Input: part model. Units: mm. Frame: model coordinates. A direction names the side the tool comes from. Give positions to 0.01 mm unless a question says otherwise; leave off trailing zeros. Loops run counter-clockwise (first coordinate to the right, second up) from the corner with the lowest first, then second, coordinate; pieces in that order, holes last. Notation, with made-up numbers: M -19,-16 L 4,-16 A17 cw 4,11 Z; hole C 24.25,-32.75 d4. An arc over 180 degrees is marked long. One line per item, written item: value. Start each with the question number.
(1) Section A-A on y = 101.6. Output: boundary loops of the cut face in (x, z) (1 decimal).
(2) Pin query (flat end, axial travel): P1, Ø10, axis at y = 119.5, z = 95.5, coming from the +X side; P2, Ø4, axis at y = 51, z = 113, coming from the -X side; P3, Ø12, axis at x = 43.5, y = 83.5, coming from the +Z side. Return the tip coordinate at first contact, or that it passes through.
(3) Section C-C on z = 101. Output: boundary loops of the cut face in (x, y) (3 decimals), plus the area to 3 significant figures.
(4) Section B-B on x = 127. Output: boundary loops of the cut face in (y, z) (3 decimals), plus the area to 3 significant figures.
(5) Section D-D on y = 54.5. Output: boundary loops of the cut face in (x, z).
(6) Pull-direction query (Y, two-part tool) for faces 1 (the cylindrical face through (117.484, 102.019, 57.95)), 2 (the flat face through (88, 0, 56)), 3 (the flat face through (88, 139.7, 56)); classes: released by +Y, released by -Y, zero draft, split by the parting line, or undercut.
(7) Access query for faces 4 (the flat face through (76.2, 69, 112)), 5 (the cylindrical face through (170.16, 132.46, 57.95)). Directions: +Z, -Z, +X, -X, +Y, -Y. A direction counts if a zero-diameter tool reaches every point of the face in a straight line with its end or side. Return the directions, or none.
(8) Ray query, line 1 along Y through (x, z) = (127, 66) (3 decimals); line 2 along X through (y, z) = (102.5, 8); line 3 along X through (y, z) = (98, 34.5). Return the intervals inside material, ascending. Write a range as from..to.
```python
from build123d import *

# Parameters (mm, degrees)
F0_W     = 177.8
F0_H     = 139.7
F1_DEPTH = 114.3
F2_W     = 76.2
F2_H     = 139.7
F3_DEPTH = 4.7625
F4_R     = 9.525
F5_DEPTH = 114.301
F6_R     = 25.4


with BuildPart() as f1:
    # F0 (on Top) → F1 (new body)
    with BuildSketch(Plane.XY):
        with Locations((88.9, 69.85)):
            Rectangle(F0_W, F0_H)
    extrude(amount=F1_DEPTH)

    # F2 (on face) → F3 (cut)
    with BuildSketch(Plane.XY.offset(114.3)):
        with Locations((38.1, 69.85)):
            Rectangle(F2_W, F2_H)
    extrude(amount=-F3_DEPTH, mode=Mode.SUBTRACT)

    # F4 (on face) → F5 (cut, through all)
    with BuildSketch(Plane.XY.offset(114.3)):
        with Locations((127, 101.6)):
            Circle(F4_R)
        with Locations((127, 38.1)):
            Circle(F4_R)
    extrude(amount=-F5_DEPTH, mode=Mode.SUBTRACT)

    # F6
    f6_edges = [f1.edges().sort_by_distance(p)[0] for p in [
        (0, 0, 54.76875),
        (177.8, 0, 57.15),
        (177.8, 139.7, 57.15),
        (0, 139.7, 54.76875),
    ]]
    fillet(f6_edges, radius=F6_R)


solid = f1.part
```
Output values:
1. outline: M 0,0 L 117.5,0 L 117.5,114.3 L 76.2,114.3 L 76.2,109.5 L 0,109.5 Z; M 136.5,0 L 177.8,0 L 177.8,114.3 L 136.5,114.3 Z
2. P1: stops at x = 177.8
2. P2: stops at x = 76.2
2. P3: stops at z = 109.54
3. outline: M 0,25.4 A25.4 ccw 25.4,0 L 152.4,0 A25.4 ccw 177.8,25.4 L 177.8,114.3 A25.4 ccw 152.4,139.7 L 25.4,139.7 A25.4 ccw 0,114.3 Z; hole C 127,38.1 d19.05; hole C 127,101.6 d19.05
3. area: 23,700 mm²
4. outline: M 0,0 L 28.575,0 L 28.575,114.3 L 0,114.3 Z; M 47.625,0 L 92.075,0 L 92.075,114.3 L 47.625,114.3 Z; M 111.125,0 L 139.7,0 L 139.7,114.3 L 111.125,114.3 Z
4. area: 11,600 mm²
5. outline: M 0,0 L 177.8,0 L 177.8,114.3 L 76.2,114.3 L 76.2,109.54 L 0,109.54 Z
6. face 1: undercut
6. face 2: released by -Y
6. face 3: released by +Y
7. face 4: +Z, -X, +Y, -Y
7. face 5: +Z, -Z, +X, +Y
8. line 1: y = 0..28.575, 47.625..92.075, 111.125..139.7
8. line 2: x = 0..117.52, 136.48..177.8
8. line 3: x = 0..118.18, 135.82..177.8
